Part model, mm, in its own coordinate system. A direction names the side the tool comes from. Round coordinates to 2 decimals unless told otherwise and drop trailing zeros. Write each loop counter-clockwise with the first axis right and the second up, starting at its lowest first coordinate (ties: lowest second). Pieces come first, ordered by that corner, then holes.
1) Saw through at C-C on y = 15.5. Write the cut outline in (x, z), and give its area (3 significant figures).
2) Drill centre lines: L1, parallel to Y at x = 0, z = 2; L2, parallel to X at y = 10, z = 38; L3, parallel to Z at x = 0.5, y = 20. Where is each one in solid material? Low to high.
3) Saw through at D-D on x = -9. Write the cut outline in (y, z).
4) Saw through at A-A on x = 0. Write the cut outline in (y, z).
5) Which spindle directions (+Z, -Z, +X, -X, +Y, -Y) get a long thin tool onto all of the face, cutting with end or side? Do faces 4 (the flat face through (-19.05, 4, 13)), 5 (the flat face through (0, 35, 6.35)), 6 (the flat face through (0, 0, 26)). Say none if no direction does.
6) Pull direction Z, two halves, no side cores. Call faces 1 (the flat face through (0, 19.05, 26)), 2 (the cylindrical face through (-0.419, 9.392, 57.145)), 3 (the cylindrical face through (1.907, 9.392, 32.043)): +Z half, -Z half, draft (parallel to the pull), parting line (faces both ways), or undercut.
7) Flat gauge pins, fed straight in: pin 1 (9.5 mm diameter, centred on x = -6.5, y = 39, fed in from +Z); pin 2 (6.5 mm diameter, centred on x = 0, y = 28.575, fed in from -Z); pin 3 (6 mm diameter, centred on x = -14.5, y = 20.5, fed in from +Z); pin 4 (3 mm diameter, centred on x = -3, z = 26.5, fed in from -Y). Where does each tip first touch, or does it go through?
8) Saw through at B-B on z = 42.5. Write the cut outline in (x, y), and give its area (3 significant figures).
```python
from build123d import *

# Parameters (mm, degrees)
SKETCH1_W           = 38.1
SKETCH1_H           = 101.6
BOSS_EXTRUDE1_DEPTH = 6.35
SKETCH2_R           = 5.5626
SKETCH2_R_2         = 5.588
CUT_EXTRUDE1_DEPTH  = 55.624765446
SKETCH3_W           = 38.1
SKETCH3_H           = 19.05
BOSS_EXTRUDE2_DEPTH = 31.75
BOSS_EXTRUDE3_DEPTH = 19.05
SKETCH5_R           = 6.35
CUT_EXTRUDE2_DEPTH  = 79.801427652


with BuildPart() as part:
    # Sketch1 → Boss-Extrude1 (new body)
    with BuildSketch(Plane.XY):
        Rectangle(SKETCH1_W, SKETCH1_H)
    extrude(amount=BOSS_EXTRUDE1_DEPTH)

    # Sketch2 → Cut-Extrude1 (cut, through all)
    with BuildSketch(Plane.XY.offset(6.35)):
        with Locations((0, 28.575)):
            Circle(SKETCH2_R)
        with Locations((0, -28.575)):
            Circle(SKETCH2_R_2)
    extrude(amount=-CUT_EXTRUDE1_DEPTH, mode=Mode.SUBTRACT)

    # Sketch3 → Boss-Extrude2 (add)
    with BuildSketch(Plane.XY.offset(6.35)):
        with Locations((0, 9.525)):
            Rectangle(SKETCH3_W, SKETCH3_H)
    extrude(amount=BOSS_EXTRUDE2_DEPTH)

    # Sketch4 → Boss-Extrude3 (add)
    with BuildSketch(Plane.XZ):
        with BuildLine():
            Line((19.05, 38.1), (-19.05, 38.1))
            ThreePointArc((-19.05, 38.1), (0, 57.15), (19.05, 38.1))
        make_face()
    extrude(amount=-BOSS_EXTRUDE3_DEPTH)

    # Sketch5 → Cut-Extrude2 (cut, through all)
    with BuildSketch(Plane.XZ):
        with Locations(Location((0, 38.1, 0), (0, 0, 270))):
            Circle(SKETCH5_R)
    extrude(amount=-CUT_EXTRUDE2_DEPTH, mode=Mode.SUBTRACT)


solid = part.part
```
Completed:
1. outline: (-19.05, 0) - (19.05, 0) - (19.05, 38.1) arc R19.05 ccw to (-19.05, 38.1) - close; hole circle Ø12.7 at (0, 38.1)
1. area: 1,890 mm2
2. L1: y = -50.8 to -34.16, -22.99 to 23.01, 34.14 to 50.8
2. L2: x = -19.05 to -6.35, 6.35 to 19.05
2. L3: z = 0 to 6.35
3. outline: (-50.8, 0) - (50.8, 0) - (50.8, 6.35) - (19.05, 6.35) - (19.05, 54.89) - (0, 54.89) - (0, 6.35) - (-50.8, 6.35) - close
4. outline: (-50.8, 0) - (-34.16, 0) - (-34.16, 6.35) - (-50.8, 6.35) - close; (-22.99, 0) - (23.01, 0) - (23.01, 6.35) - (19.05, 6.35) - (19.05, 31.75) - (0, 31.75) - (0, 6.35) - (-22.99, 6.35) - close; (0, 44.45) - (19.05, 44.45) - (19.05, 57.15) - (0, 57.15) - close; (34.14, 0) - (50.8, 0) - (50.8, 6.35) - (34.14, 6.35) - close
5. face 4: +Z, -Z, -X, +Y, -Y
5. face 5: +Z, +X, -X, +Y
5. face 6: +Z, +X, -X, -Y
6. face 1: draft
6. face 2: +Z half
6. face 3: undercut
7. pin 1: stops at z = 6.35
7. pin 2: passes through
7. pin 3: stops at z = 53
7. pin 4: stops at y = 0
8. outline: (-18.53, 0) - (-4.58, 0) - (-4.58, 19.05) - (-18.53, 19.05) - close; (4.58, 0) - (18.53, 0) - (18.53, 19.05) - (4.58, 19.05) - close
8. area: 532 mm2
